Drawing for the job (mm, zero at the part's lowest x, y, z). A direction names the side the tool comes from. Coordinates: 2 decimals unless noted, no trailing zeros. Write each loop counter-clockwise with the first axis right and the second up, starting at its lowest first coordinate (ties: lowest second). Pieces come first, ordered by that corner, then holes.
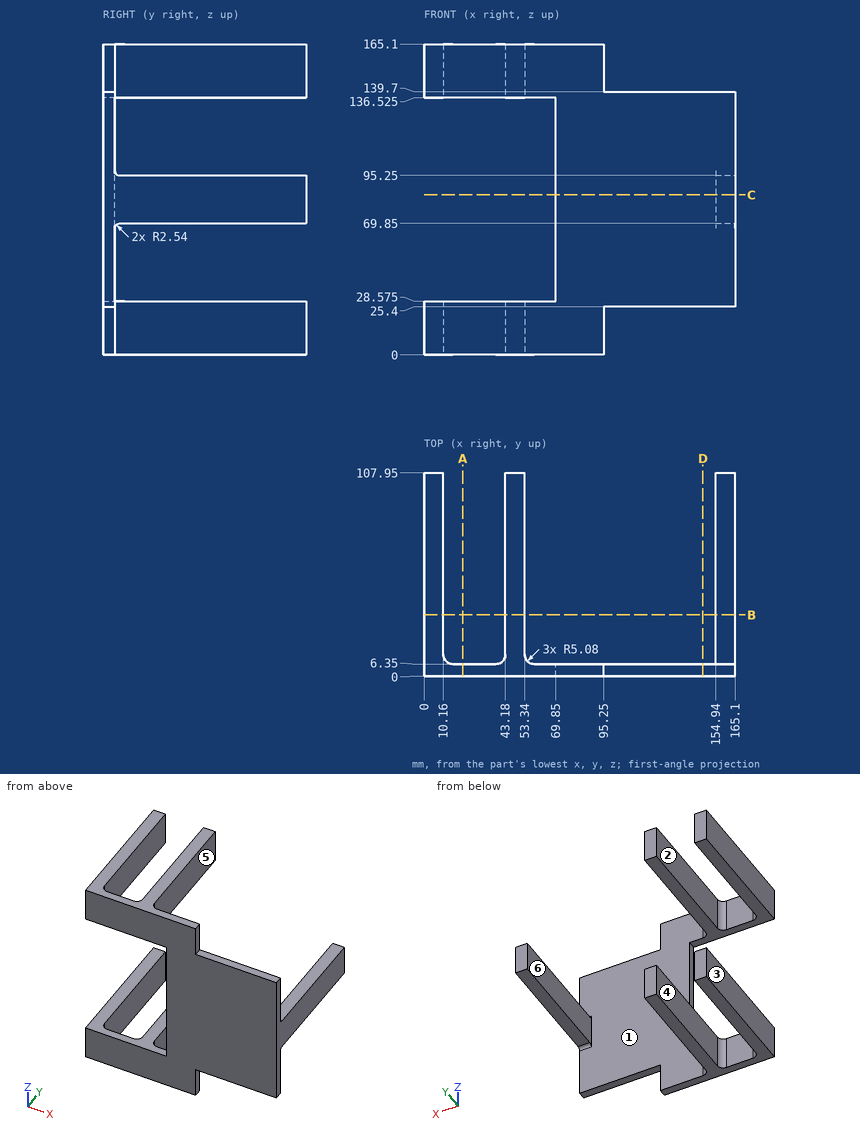
Item 1: Saw through at A-A, the plane x = 20.5. Write the cut outline in (y, z) (3 decimals).
Item 2: Wall check: line 1 along X through (y, z) = (47, 18.5); line 2 along X through (y, z) = (12.5, 79.5); line 3 along Y through (x, z) = (79.5, 60.5). Give the ranges that are in metal, low to high.
Item 3: Flat gauge pins, fed straight in: pin 1 Ø14.5 at (y, z) = (47.5, 144.5) entering from +X; pin 2 Ø7 at (y, z) = (3, 157) entering from +X; pin 3 Ø11 at (x, y) = (159, 40.5) entering from +Z; pin 4 Ø12 at (y, z) = (33, 29.5) entering from -X. Where does each tip first touch, or does it go through?
Item 4: Saw through at D-D, the plane x = 148. Write the cut outline in (y, z).
Item 5: Saw through at C-C, the plane z = 85. Write the cut outline in (x, y).
Item 6: Saw through at B-B, the plane y = 32.5. Write the cut outline in (x, z) (3 decimals), and give its area (3 significant figures).
Item 7: Two-plate mould, pull along X, no slides. Class the marked faces 1, 2 and 3: +X half, -X half, draft (parallel to the pull), parting line (faces both ways), or undercut.
Item 8: Which spindle directions (+Z, -Z, +X, -X, +Y, -Y) get a long thin tool onto all of the face, cutting with end or side? Do the marked faces 4, 5 and 6. Say none if no direction does.
Working result:
1. outline: (0, 0) - (6.35, 0) - (6.35, 28.575) - (0, 28.575) - close; (0, 136.525) - (6.35, 136.525) - (6.35, 165.1) - (0, 165.1) - close
2. line 1: x = 0 to 10.16, 43.18 to 53.34
2. line 2: x = 154.94 to 165.1
2. line 3: y = 0 to 6.35
3. pin 1: stops at x = 53.34
3. pin 2: stops at x = 95.25
3. pin 3: stops at z = 95.25
3. pin 4: stops at x = 0
4. outline: (0, 25.4) - (6.35, 25.4) - (6.35, 139.7) - (0, 139.7) - close
5. outline: (69.85, 0) - (165.1, 0) - (165.1, 107.95) - (154.94, 107.95) - (154.94, 6.35) - (69.85, 6.35) - close
6. outline: (0, 0) - (10.16, 0) - (10.16, 28.575) - (0, 28.575) - close; (0, 136.525) - (10.16, 136.525) - (10.16, 165.1) - (0, 165.1) - close; (43.18, 0) - (53.34, 0) - (53.34, 28.575) - (43.18, 28.575) - close; (43.18, 136.525) - (53.34, 136.525) - (53.34, 165.1) - (43.18, 165.1) - close; (154.94, 69.85) - (165.1, 69.85) - (165.1, 95.25) - (154.94, 95.25) - close
6. area: 1,420 mm2
7. face 1: draft
7. face 2: undercut
7. face 3: -X half
8. face 4: +Z, -Z, +Y
8. face 5: +Z, -Z, +X, +Y
8. face 6: +Z, -Z, -X, +Y
